Autodesk Inventor part; units mm, degrees
ref_plane "YZ Plane" through (0, 0, 0) normal (1, 0, 0) x (0, 1, 0)
ref_plane "XZ Plane" through (0, 0, 0) normal (0, 1, 0) x (-1, 0, 0)
ref_plane "XY Plane" through (0, 0, 0) normal (0, 0, 1) x (1, 0, 0)
sketch "스케치1" plane through (0, 0, 0) normal (0, 1, 0) x (-1, 0, 0)
  circle A0 centre (0, 0) radius 2
  line L0 (0, 0) -> (0, -45)
  line L1 (23, -45) -> (-23, -45)
  circle A1 centre (23, -45) radius 2
  circle A2 centre (-23, -45) radius 2
  circle A3 centre (23, -45) radius 10
  circle A4 centre (-23, -45) radius 10
  circle A5 centre (0, 0) radius 10
  arc A6 (9.447, -3.2795) -> (25.8755, -35.4224) centre (33.0643, -11.4782) ccw
  line L2 (0, -115.952) -> (0, 30.992)
  arc A7 (-25.8755, -35.4224) -> (-9.447, -3.2795) centre (-33.0643, -11.4782) ccw
  arc A8 (18.8182, -54.0836) -> (-18.8182, -54.0836) centre (0, -94.96) ccw
  point P0 (-9.447, -3.2795)
  point P1 (-25.8755, -35.4224)
  dimension "d6" = 20
  dimension "d7" = 20
  dimension "d0" = 4
  dimension "d1" = 45
  dimension "d2" = 46
  dimension "d3" = 4
  dimension "d4" = 4
  dimension "d5" = 20
  dimension "d8" = 25
  dimension "d9" = 45
extrude "돌출1" add sketch "스케치1" along normal blind 5 contours A0 L2 A5 L0 | A0 L0 A5 L2 | A5 A6 A3 L1 L0 | L0 L1 A4 A7 A5 | L2 A8 A4 L1 | L1 A3 A8 L2 | A4 | A3
sketch "스케치2" plane through (0, 5, 0) normal (0, 1, 0) x (1, 0, 0)
  arc A0 (-9.447, 3.2795) -> (9.447, 3.2795) centre (0, 0) ccw
  arc A1 (25.8755, 35.4224) -> (9.447, 3.2795) centre (33.0643, 11.4782) ccw
  arc A2 (25.8755, 35.4224) -> (18.8182, 54.0836) centre (23, 45) ccw
  arc A3 (-18.8182, 54.0836) -> (18.8182, 54.0836) centre (0, 94.96) ccw
  arc A4 (-18.8182, 54.0836) -> (-25.8755, 35.4224) centre (-23, 45) ccw
  arc A5 (-9.447, 3.2795) -> (-25.8755, 35.4224) centre (-33.0643, 11.4782) ccw
  circle A6 centre (-23, 45) radius 2
  circle A7 centre (23, 45) radius 2
  circle A8 centre (0, 0) radius 2
  circle A9 centre (-23, 45) radius 4
  circle A10 centre (23, 45) radius 4
  circle A11 centre (0, 0) radius 4
  dimension "d12" = 8
  dimension "d13" = 8
  dimension "d14" = 8
extrude "돌출2" add sketch "스케치2" along normal blind 2 contours A5 A4 A3 A2 A1 A0
sketch "스케치7" plane through (0, 0, 0) normal (1, 0, 0) x (0, 1, 0)
  line L0 (5, -43) -> (5, -47)
  line L1 (0, -43) -> (0, -47)
  line L2 (7, -41) -> (7, -49)
  line L3 (5, -49) -> (5, -41)
  line L4 (0, -45) -> (7, -45)
  line L5 (7, -41) -> (7, -49)
  line L6 (7, -45) -> (0, -45)
  line L7 (7, -55) -> (7, -35.4224)
  line L8 (0, -49.96) -> (0, -54.0836)
  line L9 (0, -45) -> (0, -49.96)
  line L10 (0, -49.96) -> (70, -150)
  line L11 (77, -147.7942) -> (8.6259, -50.0779)
  arc A0 (7, -44.9181) -> (8.6259, -50.0779) centre (16, -44.9181) ccw
  line L12 (77, -147.7942) -> (77, -210)
  line L13 (70, -150) -> (70, -210)
  line L14 (77, -210) -> (70, -210)
  line L15 (77, -210) -> (85, -210)
  line L16 (85, -210) -> (85, -173.1814)
  arc A1 (85, -173.1814) -> (77, -147.7942) centre (40.718, -173.1814) ccw
  point P0 (0, 0)
  point P1 (7, -54.0836)
  point P2 (7, -44.9181)
  dimension "d34" = 7
  dimension "d35" = 9
  dimension "d36" = 7
  dimension "d37" = 60
  dimension "d39" = 165
  dimension "d40" = 70
  dimension "d41" = 8
extrude "돌출7" add sketch "스케치7" along normal mid plane 38
sketch "스케치8" plane through (19, 85, -210) normal (0, 0, -1) x (-1, 0, 0)
  line L0 (38, -15) -> (0, -15)
  line L1 (19, -15) -> (19, -8)
  line L2 (38, -8) -> (0, -8)
  line L3 (9, -10) -> (29, -10)
  circle A0 centre (9, -10) radius 2
  circle A1 centre (29, -10) radius 2
  line L4 (38, 0) -> (0, 0)
  point P0 (19, -85)
  point P1 (19, -10)
  dimension "d44" = 20
  dimension "d45" = 4
  dimension "d46" = 4
  dimension "d47" = 10
extrude "돌출8" cut sketch "스케치8" against normal blind 25 contours A0 | A1
properties part number "라이다 고"
Input: part model. Units: mm. Frame: model coordinates. A direction names the side the tool comes from. Round coordinates to 2 decimals unless told otherwise and drop trailing zeros. Write each loop counter-clockwise with the first axis right and the second up, starting at its lowest first coordinate (ties: lowest second). Pieces come first, ordered by that corner, then holes. Notation, with made-up numbers: (18, 41.5) -> (51, 41.5) arc R32 cw to (51, 80.5) -> close; hole circle Ø2 at (41, 7). An arc over 180 degrees is marked (long way). Answer as CSV lines item,"result".
1. Contact query for flat-ended pins moving along their axis: P1, Ø1.5, axis at x = -1.5, y = 63, coming from the -Z side; P2, Ø6.5, axis at x = -23, z = -45, coming from the +Y side; P3, Ø3, axis at x = 10, y = 75, coming from the +Z side; P4, Ø4, axis at y = 66.5, z = -157, coming from the +X side. Output: stop coordinate, or through.
Geometry says:
P1,"stops at z = -141.07"
P2,"stops at y = 5"
P3,"stops at z = -142.79"
P4,"passes through"
2. Ray query, L1, parallel to X at y = 5.4, z = -45; L2, parallel to Z at x = 0, y = 3.55; L3, parallel to Y at x = -5.5, z = -27.5. Return the intervals inside material, ascending. Write a range as [from, to].
Geometry says:
L1,"x = [-33, -27], [-19, 19], [27, 33]"
L2,"z = [-55.03, -2], [2, 10]"
L3,"y = [0, 7]"
3. Section D-D (x = -14). Return the cut outline in (y, z).
Geometry says:
outline,"(0, -52.19) -> (1.56, -52.19) -> (70, -150) -> (70, -210) -> (85, -210) -> (85, -173.18) arc R44.28 ccw to (77, -147.79) -> (8.63, -50.08) arc R9 cw to (7, -45) -> (7, -27.65) -> (0, -27.65) -> close"
4. Reachability of faces 1 (the flat face through (0, 70, -180)), 2 (the cylindrical face through (14.537, 0.688, -52.373)), 3 (the flat face through (2, 5, -1)) from +Z, -Z, +X, -X, +Y, -Y: full face, straight path, thin tool, end or side. Return the list, or none.
Geometry says:
face 1,"-Z, +X, -X, -Y"
face 2,"-Z, -Y"
face 3,"+Y"
5. Section B-B (y = 75). Return the cut outline in (x, z), plus the area to 3 significant figures.
Geometry says:
outline,"(-19, -210) -> (-12, -210) -> (-12, -185) -> (-8, -185) -> (-8, -210) -> (8, -210) -> (8, -185) -> (12, -185) -> (12, -210) -> (19, -210) -> (19, -144.94) -> (-19, -144.94) -> close"
area,"2,270 mm^2"
6. Section A-A (x = -23). Return the cut outline in (y, z).
Geometry says:
outline,"(0, -55) -> (7, -55) -> (7, -49) -> (5, -49) -> (5, -47) -> (0, -47) -> close; (0, -43) -> (5, -43) -> (5, -41) -> (7, -41) -> (7, -34.36) -> (0, -34.36) -> close"
7. Section C-C (z = -14). Return the cut outline in (x, y).
Geometry says:
outline,"(-8.19, 0) -> (8.19, 0) -> (8.19, 7) -> (-8.19, 7) -> close"
8. Mould query, pull axis X, two halves, no side actions, for faces 4 (the flat face through (0, 7, -30)), 5 (the cylindrical face through (-10, 77, -198)), 6 (the cylindrical face through (-10.933, 3.451, -23.107)). Classes: +X half, -X half, draft (parallel to the pull), parting line (faces both ways), or undercut.
Geometry says:
face 4,"draft"
face 5,"undercut"
face 6,"-X half"
